Model file for the job. Use its own axes, mm. Face numbers are marked on the shaded views. A direction names the side the tool comes from. Coordinates: 2 decimals unless noted, no trailing zeros. Write each loop counter-clockwise with the first axis right and the second up, starting at its lowest first coordinate (ties: lowest second). Pieces come first, ordered by that corner, then holes. Notation, with made-up numbers: M 8,61 L 24,61 A25 ccw 24,85 Z; hole C 34,51 d1. An arc over 180 degrees is marked long. Use CSV: the item, a comma, the result in double quotes. Start each with the question number.
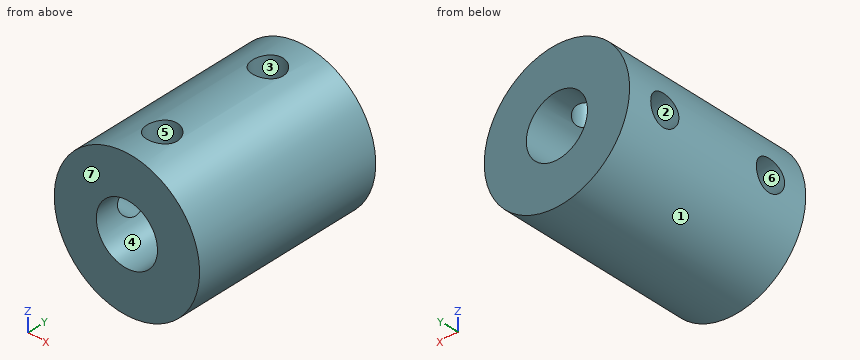
from build123d import *

# Parameters (mm, degrees)
SKETCH1_R           = 9.5
BOSS_EXTRUDE1_DEPTH = 25
SKETCH2_R           = 4
CUT_EXTRUDE1_DEPTH  = 25
SKETCH3_R           = 2
CUT_EXTRUDE2_DEPTH  = 10
SKETCH4_R           = 2
CUT_EXTRUDE3_DEPTH  = 10


with BuildPart() as part:
    # Sketch1 → Boss-Extrude1 (new body)
    with BuildSketch(Plane(origin=(0, 0, 0), x_dir=(1, 0, 0), z_dir=(0, 1, 0))):
        with Locations(Location((0, 0, 0), (0, 0, 270))):
            Circle(SKETCH1_R)
    extrude(amount=BOSS_EXTRUDE1_DEPTH)

    # Sketch2 → Cut-Extrude1 (cut)
    with BuildSketch(Plane(origin=(0, 25, 0), x_dir=(1, 0, 0), z_dir=(0, 1, 0))):
        with Locations(Location((0, 0, 0), (0, 0, 270))):
            Circle(SKETCH2_R)
    extrude(amount=-CUT_EXTRUDE1_DEPTH, mode=Mode.SUBTRACT)

    # Sketch3 → Cut-Extrude2 (cut)
    with BuildSketch(Plane.XY):
        with Locations(Location((0, 20, 0), (0, 0, 270))):
            Circle(SKETCH3_R)
        with Locations(Location((0, 5, 0), (0, 0, 270))):
            Circle(SKETCH3_R)
    extrude(amount=CUT_EXTRUDE2_DEPTH, mode=Mode.SUBTRACT)

    # Sketch4 → Cut-Extrude3 (cut)
    with BuildSketch(Plane(origin=(0, 0, 0), x_dir=(0, 0, -1), z_dir=(1, 0, 0))):
        with Locations((0, 20)):
            Circle(SKETCH4_R)
        with Locations((0, 5)):
            Circle(SKETCH4_R)
    extrude(amount=-CUT_EXTRUDE3_DEPTH, mode=Mode.SUBTRACT)


solid = part.part
1) Wall check: L1, parallel to Y at x = 0, z = 6.25; L2, parallel to Y at x = 1.25, z = 4.5; L3, parallel to X at y = 16, z = 0. Give the ranges that are in metal, low to high. Write a range as [from, to].
2) Band-saw the part on B-B on z = 0. List the corners of the cut face in (x, y).
3) Band-saw the part on D-D on z = 8. List the corners of the cut face in (x, y), then the cut area to 3 significant figures.
4) Two-plate mould, pull along Z, no slides. Class the marked faces 1, 2, 3 and 4: pulls with the +Z half, pulls with the -Z half, needs draft (parallel to the pull), parting line crosses it, or undercut.
5) Band-saw the part on C-C on y = 21. List the corners of the cut face in (x, z).
6) Tool access for the marked faces 5, 6 and 7: list every direction of +Z, -Z, +X, -X, +Y, -Y with a clear straight run to the whole face (end or side of a thin tool).
7) Drop flat-ended pins along their axis: P1, Ø6, axis at x = 7, y = 12.5, coming from the +Z side; P2, Ø3.5, axis at y = 20, z = 0, coming from the -X side; P3, Ø8, axis at x = -4.5, y = 3.5, coming from the +Z side; P4, Ø6.5, axis at x = 0, z = 0, coming from the -Y side. Give the stop position or say it passes through.
8) Band-saw the part on A-A on x = 0. List the corners of the cut face in (y, z).
Findings below:
1,L1,"y = [0, 3], [7, 18], [22, 25]"
1,L2,"y = [0, 3.44], [6.56, 18.44], [21.56, 25]"
1,L3,"x = [-9.5, -4], [4, 9.5]"
2,outline,"M -9.5,0 L -4,0 L -4,3 L -9.5,3 Z; M -9.5,7 L -4,7 L -4,18 L -9.5,18 Z; M -9.5,22 L -4,22 L -4,25 L -9.5,25 Z; M 4,0 L 9.5,0 L 9.5,25 L 4,25 Z"
3,outline,"M -5.12,0 L 5.12,0 L 5.12,25 L -5.12,25 Z; hole C 0,5 d4; hole C 0,20 d4"
3,area,"231 mm2"
4,face 1,"parting line crosses it"
4,face 2,"undercut"
4,face 3,"needs draft"
4,face 4,"undercut"
5,outline,"M -9.34,-1.73 A9.5 ccw long 1.73,9.34 L 1.73,3.61 A4 cw long -3.61,-1.73 Z; M -9.34,1.73 L -3.61,1.73 A4 cw -1.73,3.61 L -1.73,9.34 A9.5 ccw Z"
6,face 5,"+Z"
6,face 6,"-X"
6,face 7,"+Z, -Z, +X, -X, -Y"
7,P1,"stops at z = 8.62"
7,P2,"stops at x = 3.6"
7,P3,"stops at z = 9.49"
7,P4,"passes through"
8,outline,"M 0,-9.5 L 25,-9.5 L 25,-4 L 0,-4 Z; M 0,4 L 3,4 L 3,9.5 L 0,9.5 Z; M 7,4 L 18,4 L 18,9.5 L 7,9.5 Z; M 22,4 L 25,4 L 25,9.5 L 22,9.5 Z"
